Part model, mm, in its own coordinate system. A direction names the side the tool comes from. Round coordinates to 2 decimals unless told otherwise and drop trailing zeros. Loops run counter-clockwise (first coordinate to the right, second up) from the corner with the lowest first, then second, coordinate; pieces in that order, holes last.
from build123d import *

# Parameters (mm, degrees)
SKETCH_2_W          = 6.5
SKETCH_2_H          = 8
CUT_EXTRUDE_1_DEPTH = 3


with BuildPart() as part:
    # Sketch 1 → Revolve 1 (revolve)
    with BuildSketch(Plane.XY, mode=Mode.PRIVATE) as revolve_1_sk:
        Polygon((-10, 1.5), (-9.8645, 1.3645), (-0.1355, 1.3645), (0, 1.5), (0, 3), (-7, 3), (-7, 4), (-9.5, 4), (-10, 3.5), align=None)
    revolve(revolve_1_sk.sketch.rotate(Axis((0, 0, 0), (-1, 0, 0)), 270), axis=Axis((0, 0, 0), (-1, 0, 0)))

    # Sketch 2 → Cut-Extrude 1 (cut)
    with BuildSketch(Plane(origin=(0, 2.5, 0), x_dir=(1, 0, 0), z_dir=(0, 1, 0))):
        with Locations((-3.25, 0)):
            Rectangle(SKETCH_2_W, SKETCH_2_H)
    extrude(amount=CUT_EXTRUDE_1_DEPTH, mode=Mode.SUBTRACT)

    # Sketch 3 → Cut-Revolve 1 (revolve, cut)
    with BuildSketch(Plane.XY, mode=Mode.PRIVATE) as cut_revolve_1_sk:
        Polygon((-0.25, 3), (0, 2.75), (0, 3), align=None)
    revolve(cut_revolve_1_sk.sketch.rotate(Axis((0, 0, 0), (-1, 0, 0)), 270), axis=Axis((0, 0, 0), (-1, 0, 0)), mode=Mode.SUBTRACT)


solid = part.part
1) Drop flat-ended pins along their axis: pin 1 Ø2 at (x, y) = (-2, 2.5) entering from -Z; pin 2 Ø2 at (x, z) = (-4.5, -1) entering from +Y. Give the stop position or say it passes through.
Values:
pin 1: stops at z = -2.6
pin 2: stops at y = 2.5
2) Slice it at C-C, the plane x = -5.5. Give the cut face in (y, z), then the cut area to 3 significant figures.
Values:
outline: (2.5, -1.66) - (2.5, 1.66) arc R3 ccw (long way) to start; hole circle Ø2.73 at (0, 0)
area: 21.3 mm2
3) Wall check: line 1 along Y through (x, z) = (-2, 0); line 2 along X through (y, z) = (0.25, 3.25); line 3 along Y through (x, z) = (-5.75, 0.75). Give the ranges that are in metal, low to high.
Values:
line 1: y = -3 to -1.36, 1.36 to 2.5
line 2: x = -10 to -7
line 3: y = -2.9 to -1.14, 1.14 to 2.5
4) Mould opens along Z. For faces 3 (the face through (-3, 2.5, 0)), 4 (the face through (-4.93, -0.52, 1.26)), 5 (the face through (-3.67, -2.93, -0.65)) say: released by +Z, released by -Z, zero draft, split by the parting line, or undercut.
Values:
face 3: zero draft
face 4: undercut
face 5: split by the parting line
5) Slice it at B-B, the plane y = 0. Give the cut face in (x, z), then the cut area to 3 significant figures.
Values:
outline: (-10, -3.5) - (-9.5, -4) - (-7, -4) - (-7, -3) - (-0.25, -3) - (0, -2.75) - (0, -1.5) - (-0.14, -1.36) - (-9.86, -1.36) - (-10, -1.5) - close; (-10, 1.5) - (-9.86, 1.36) - (-0.14, 1.36) - (0, 1.5) - (0, 2.75) - (-0.25, 3) - (-7, 3) - (-7, 4) - (-9.5, 4) - (-10, 3.5) - close
area: 38.4 mm2
6) Slice it at A-A, the plane z = 0. Give the cut face in (x, y), then the cut area to 3 significant figures.
Values:
outline: (-10, -3.5) - (-9.5, -4) - (-7, -4) - (-7, -3) - (-0.25, -3) - (0, -2.75) - (0, -1.5) - (-0.14, -1.36) - (-9.86, -1.36) - (-10, -1.5) - close; (-10, 1.5) - (-9.86, 1.36) - (-0.14, 1.36) - (0, 1.5) - (0, 2.5) - (-6.5, 2.5) - (-6.5, 3) - (-7, 3) - (-7, 4) - (-9.5, 4) - (-10, 3.5) - close
area: 35.1 mm2
7) Tool access for faces 1 (the face through (-7, 3, -1)), 2 (the face through (-10, -2, 0)): list every direction of +Z, -Z, +X, -X, +Y, -Y with a clear straight run to the whole face (end or side of a thin tool).
Values:
face 1: +X
face 2: +Z, -Z, -X, +Y, -Y
